from build123d import *

# Parameters (mm, degrees)
SKETCH1_R           = 6.5
SKETCH1_R_2         = 2.5
BOSS_EXTRUDE1_DEPTH = 3
SKETCH1_3_R         = 11.5
SKETCH1_3_R_2       = 6.5
SKETCH1_3_R_3       = 1.5
BOSS_EXTRUDE2_DEPTH = 8
SKETCH1_4_R         = 11.5
BOSS_EXTRUDE3_DEPTH = 15
SKETCH1_5_R         = 2.5
BOSS_EXTRUDE4_DEPTH = 20
SKETCH3_W           = 174
SKETCH3_H           = 78
SKETCH3_R           = 11.5
CUT_EXTRUDE1_DEPTH  = 5


with BuildPart() as part:
    # Sketch1 → Boss-Extrude1 (new body)
    with BuildSketch(Plane(origin=(0, 0, 0), x_dir=(1, 0, 0), z_dir=(0, 1, 0))):
        with Locations(Location((0, 0, 0), (0, 0, 270))):
            Circle(SKETCH1_R)
        with Locations(Location((0, 0, 0), (0, 0, 270))):
            Circle(SKETCH1_R_2, mode=Mode.SUBTRACT)
    extrude(amount=BOSS_EXTRUDE1_DEPTH)



with BuildPart() as body_2:
    # Sketch1_3 → Boss-Extrude2 (new body)
    with BuildSketch(Plane(origin=(0, 0, 0), x_dir=(1, 0, 0), z_dir=(0, 1, 0))):
        with Locations(Location((0, 0, 0), (0, 0, 270))):
            Circle(SKETCH1_3_R)
        with Locations(Location((0, 0, 0), (0, 0, 270))):
            Circle(SKETCH1_3_R_2, mode=Mode.SUBTRACT)
        with Locations(Location((0, 9, 0), (0, 0, 270))):
            Circle(SKETCH1_3_R_3, mode=Mode.SUBTRACT)
        with Locations(Location((9, 0, 0), (0, 0, 270))):
            Circle(SKETCH1_3_R_3, mode=Mode.SUBTRACT)
        with Locations(Location((0, -9, 0), (0, 0, 270))):
            Circle(SKETCH1_3_R_3, mode=Mode.SUBTRACT)
        with Locations(Location((-9, 0, 0), (0, 0, 270))):
            Circle(SKETCH1_3_R_3, mode=Mode.SUBTRACT)
    extrude(amount=BOSS_EXTRUDE2_DEPTH)


with BuildPart() as part_1:
    add(part.part)

    add(body_2.part)  # Boss-Extrude3 merges body 2
    # Sketch1_4 → Boss-Extrude3 (add)
    with BuildSketch(Plane(origin=(0, 0, 0), x_dir=(1, 0, 0), z_dir=(0, 1, 0))):
        with BuildLine():
            ThreePointArc((39.5859375, 32.942427844), (36.735072586, 36.094105365), (33.634060118, 39))
            Line((33.634060118, 39), (-33.634060118, 39))
            ThreePointArc((-33.634060118, 39), (-36.735072586, 36.094105365), (-39.5859375, 32.942427844))
            ThreePointArc((-39.5859375, 32.942427844), (-21.147829464, 20.855717142), (-14, 0))
            ThreePointArc((-14, 0), (-21.147829464, -20.855717142), (-39.5859375, -32.942427844))
            ThreePointArc((-39.5859375, -32.942427844), (-36.735072586, -36.094105365), (-33.634060118, -39))
            Line((-33.634060118, -39), (33.634060118, -39))
            ThreePointArc((33.634060118, -39), (36.735072586, -36.094105365), (39.5859375, -32.942427844))
            ThreePointArc((39.5859375, -32.942427844), (14, 0), (39.5859375, 32.942427844))
        make_face()
        with Locations(Location((0, 0, 0), (0, 0, 270))):
            Circle(SKETCH1_4_R, mode=Mode.SUBTRACT)
    extrude(amount=BOSS_EXTRUDE3_DEPTH)

    # Sketch1_5 → Boss-Extrude4 (add)
    # profile 1 of 2: a face of its own
    with BuildSketch(Plane(origin=(0, 0, 0), x_dir=(1, 0, 0), z_dir=(0, 1, 0))):
        with BuildLine():
            ThreePointArc((-39.5859375, 32.942427844), (-36.735072586, 36.094105365), (-33.634060118, 39))
            Line((-33.634060118, 39), (-87, 39))
            Line((-87, 39), (-87, -39))
            Line((-87, -39), (-33.634060118, -39))
            ThreePointArc((-33.634060118, -39), (-36.735072586, -36.094105365), (-39.5859375, -32.942427844))
            ThreePointArc((-39.5859375, -32.942427844), (-82, 0), (-39.5859375, 32.942427844))
        make_face()
        with Locations(Location((-79.5, -31.5, 0), (0, 0, 270))):
            Circle(SKETCH1_5_R, mode=Mode.SUBTRACT)
        with Locations(Location((-79.5, 31.5, 0), (0, 0, 270))):
            Circle(SKETCH1_5_R, mode=Mode.SUBTRACT)
    # profile 2 of 2: a face of its own
    with BuildSketch(Plane(origin=(0, 0, 0), x_dir=(1, 0, 0), z_dir=(0, 1, 0))):
        with BuildLine():
            Line((87, -39), (87, 39))
            Line((87, 39), (33.634060118, 39))
            ThreePointArc((33.634060118, 39), (36.735072586, 36.094105365), (39.5859375, 32.942427844))
            ThreePointArc((39.5859375, 32.942427844), (68.855717142, 26.852170536), (82, 0))
            ThreePointArc((82, 0), (68.855717142, -26.852170536), (39.5859375, -32.942427844))
            ThreePointArc((39.5859375, -32.942427844), (36.735072586, -36.094105365), (33.634060118, -39))
            Line((33.634060118, -39), (87, -39))
        make_face()
        with Locations(Location((79.5, -31.5, 0), (0, 0, 270))):
            Circle(SKETCH1_5_R, mode=Mode.SUBTRACT)
        with Locations(Location((79.5, 31.5, 0), (0, 0, 270))):
            Circle(SKETCH1_5_R, mode=Mode.SUBTRACT)
    extrude(amount=BOSS_EXTRUDE4_DEPTH)

    # Sketch3 → Cut-Extrude1 (cut)
    with BuildSketch(Plane.XZ):
        Rectangle(SKETCH3_W, SKETCH3_H)
        with Locations(Location((0, 0, 0), (0, 0, 90))):
            Circle(SKETCH3_R, mode=Mode.SUBTRACT)
    extrude(amount=-CUT_EXTRUDE1_DEPTH, mode=Mode.SUBTRACT)


solid = part_1.part
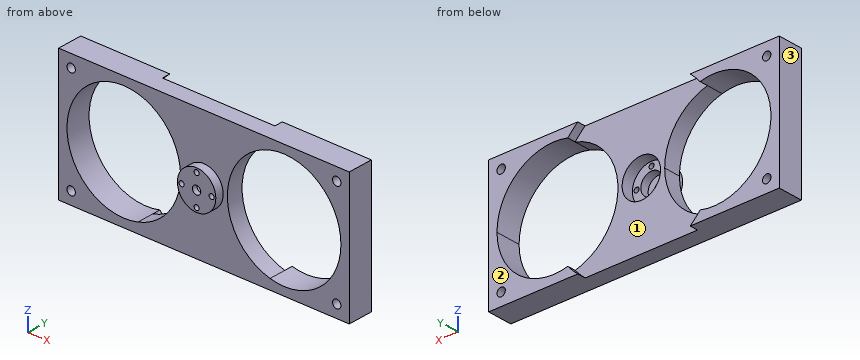
Input: part model. Units: mm. Frame: model coordinates. Face numbers are marked on the shaded views. Coordinates: 2 decimals unless noted, no trailing zeros. Loops run counter-clockwise (first coordinate to the right, second up) from the corner with the lowest first, then second, coordinate; pieces in that order, holes last.
Q1. Cut plane A-A (y = 16.75). Output: boundary loops of the cut face in (x, z), then the cut area to 3 significant figures.
Q2. Draft query along X for the marked faces 1, 2 and 3. Return one class per face: +X half, -X half, draft (parallel to the pull), parting line (faces both ways), or undercut.
Q3. Material intervals for line 1 (X direction, y = 6.75, z = 11); line 2 (X direction, y = 8.5, z = -13.5); line 3 (X direction, y = 4.4, z = 0), sorted ascending.
Q4. Contact query for flat-ended pins moving along their axis: pin 1 (3.5 mm diameter, centred on x = 9, z = 0, fed in from +Y); pin 2 (1 mm diameter, centred on y = 2.5, z = 3.5, fed in from +X); pin 3 (6 mm diameter, centred on x = 8, z = 22, fed in from -Y). Output: stop coordinate, or through.
Q5. Cut plane B-B (x = 64). Output: boundary loops of the cut face in (y, z), then the cut area to 3 significant figures.
Q6. Cut plane C-C (z = 20). Output: boundary loops of the cut face in (x, y), then the cut area to 3 significant figures.
Q7. Cut plane D-D (x = -79.5). Output: boundary loops of the cut face in (y, z), then the cut area to 3 significant figures.
Working result:
1. outline: (-87, -39) - (-33.63, -39) arc R51.5 cw to (-39.59, -32.94) arc R34 cw (long way) to (-39.59, 32.94) arc R51.5 cw to (-33.63, 39) - (-87, 39) - close; (33.63, -39) - (87, -39) - (87, 39) - (33.63, 39) arc R51.5 cw to (39.59, 32.94) arc R34 cw (long way) to (39.59, -32.94) arc R51.5 cw to start; hole circle Ø5 at (-79.5, -31.5); hole circle Ø5 at (-79.5, 31.5); hole circle Ø5 at (79.5, -31.5); hole circle Ø5 at (79.5, 31.5)
1. area: 2,620 mm2
2. face 1: undercut
2. face 2: draft
2. face 3: -X half
3. line 1: x = -87 to -80.17, -15.83 to 15.83, 80.17 to 87
3. line 2: x = -87 to -79.2, -16.8 to 16.8, 79.2 to 87
3. line 3: x = -11.5 to -10.5, -7.5 to -6.5, 6.5 to 7.5, 10.5 to 11.5
4. pin 1: stops at y = 8
4. pin 2: stops at x = 11.1
4. pin 3: stops at y = 5
5. outline: (5, -39) - (20, -39) - (20, -30) - (5, -30) - close; (5, 30) - (20, 30) - (20, 39) - (5, 39) - close
5. area: 270 mm2
6. outline: (-87, 5) - (-75.5, 5) - (-75.5, 20) - (-87, 20) - close; (-20.5, 5) - (20.5, 5) - (20.5, 15) - (-20.5, 15) - close; (75.5, 5) - (87, 5) - (87, 20) - (75.5, 20) - close
6. area: 755 mm2
7. outline: (5, -39) - (20, -39) - (20, -34) - (5, -34) - close; (5, -29) - (20, -29) - (20, -12.8) - (5, -12.8) - close; (5, 12.8) - (20, 12.8) - (20, 29) - (5, 29) - close; (5, 34) - (20, 34) - (20, 39) - (5, 39) - close
7. area: 636 mm2
